Part model, mm, in its own coordinate system. Round coordinates to 2 decimals unless told otherwise and drop trailing zeros. Loops run counter-clockwise (first coordinate to the right, second up) from the corner with the lowest first, then second, coordinate; pieces in that order, holes last. Notation, with made-up numbers: M 27,-13.75 L 79,-13.75 A16 ccw 79,3.25 Z; hole C 58,-27 d7. An arc over 180 degrees is marked long. Answer as CSV lines item,"result". Start each with the question number.
Item 1: Drop a flat-ended pin along its axis: pin 1 Ø12 at (x, y) = (12, 38.5) entering from +Z. Give the stop position or say it passes through.
Item 2: Wall check: line 1 (X direction, y = 36.5, z = 123); line 2 (X direction, y = 0.55, z = 266.7); line 3 (Y direction, x = 16.75, z = 263.5). Give the ranges that are in metal, low to high.
Item 3: Band-saw the part on A-A (y = 25.4). Count the separate pieces of the cut face and the enclosed holes in it, and give its area (3 significant figures).
Item 4: Band-saw the part on B-B (z = 227). Give the cut face in (x, y), and give its area (3 significant figures).
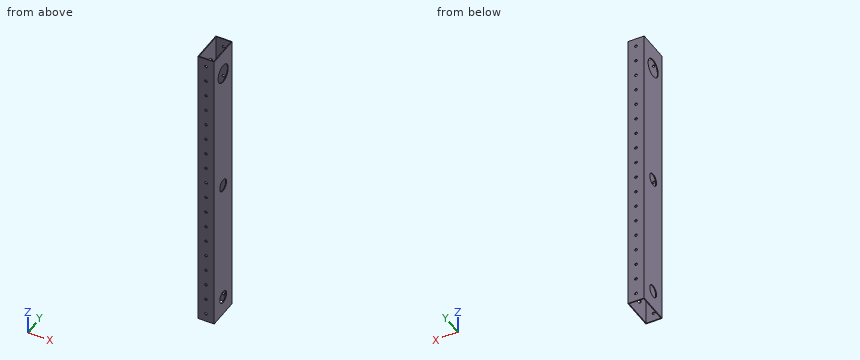
Autodesk Inventor part; units mm, degrees
ref_plane "YZ Plane" through (0, 0, 0) normal (1, 0, 0) x (0, 1, 0)
ref_plane "XZ Plane" through (0, 0, 0) normal (0, 1, 0) x (-1, 0, 0)
ref_plane "XY Plane" through (0, 0, 0) normal (0, 0, 1) x (1, 0, 0)
sketch "Sketch1" plane through (0, 0, 0) normal (0, 0, 1) x (1, 0, 0)
  line L0 (0, 0) -> (25.4, 0)
  line L1 (25.4, 0) -> (25.4, 50.8)
  line L2 (25.4, 50.8) -> (0, 50.8)
  line L3 (0, 50.8) -> (0, 0)
  line L4 (1.27, 1.27) -> (24.13, 1.27)
  line L5 (24.13, 1.27) -> (24.13, 49.53)
  line L6 (24.13, 49.53) -> (1.27, 49.53)
  line L7 (1.27, 49.53) -> (1.27, 1.27)
  dimension "d0" = 25.4
  dimension "d1" = 50.8
  dimension "d4" = 1.27
  dimension "d5" = 1.27
extrude "Extrusion1" add sketch "Sketch1" along normal blind 457.2
sketch "Sketch2" plane through (0, 50.8, 0) normal (0, 1, 0) x (1, 0, 0)
  line L0 (1.27, -457.2) -> (24.13, -457.2)
  circle A0 centre (12.7, -12.7) radius 2.0701
  line L1 (0, 0) -> (0, -457.2)
  line L2 (25.4, 0) -> (0, 0)
  dimension "d9" = 4.1402
  dimension "d10" = 12.7
  dimension "d11" = 12.7
extrude "Extrusion2" cut sketch "Sketch2" against normal blind 457.2
pattern_linear "Rectangular Pattern1" count 18 spacing 25.4 along (0, 0, 1) of "Extrusion2"
sketch "Sketch3" plane through (25.4, 0, 0) normal (1, 0, 0) x (0, 0, -1)
  line L0 (-457.2, 0) -> (-457.2, 50.8)
  line L1 (-457.2, 25.4) -> (0, 25.4) construction
  circle A0 centre (-419.1, 25.4) radius 14.2875
  circle A1 centre (-224.282, 25.4) radius 9.525
  circle A2 centre (-29.464, 25.4) radius 9.525
  point P0 (0, 0)
  dimension "d17" = 19.05
  dimension "d18" = 38.1
  dimension "d19" = 28.575
  dimension "d20" = 194.818
  dimension "d21" = 194.818
extrude "Extrusion3" cut sketch "Sketch3" against normal through all
equation "\"d0\" = u1"
equation "\"d1\" = u2"
equation "\"d4\" = u3"
equation "\"d5\" = u3"
equation "\"d6\" = u4"
equation "\"d9\" = u5"
equation "\"d10\" = u6"
equation "\"d11\" = u7"
equation "\"d12\" = u4"
equation "\"d20\" = u10"
equation "\"d21\" = u10"
equation "\"d16\" = u9"
equation "\"u1\" = 25.4"
equation "\"u2\" = 50.8"
equation "\"u3\" = 1.27"
equation "\"u4\" = 457.2"
equation "\"u5\" = 4.1402"
equation "\"u6\" = 12.7"
equation "\"u7\" = 12.7"
equation "\"u9\" = 25.4"
equation "\"u10\" = 194.818"
properties part number "VerseFrame 18in Uptake"
Answer block:
1,pin 1,"passes through"
2,line 1,"x = 0 to 1.27, 24.13 to 25.4"
2,line 2,"x = 0 to 10.63, 14.77 to 25.4"
2,line 3,"y = 0 to 1.27, 49.53 to 50.8"
3,separate pieces,"8"
3,enclosed holes,"0"
3,area,"992 mm^2"
4,outline,"M 0,0 L 25.4,0 L 25.4,16.27 L 24.13,16.27 L 24.13,1.27 L 1.27,1.27 L 1.27,16.27 L 0,16.27 Z; M 0,34.53 L 1.27,34.53 L 1.27,49.53 L 24.13,49.53 L 24.13,34.53 L 25.4,34.53 L 25.4,50.8 L 0,50.8 Z"
4,area,"141 mm^2"
